For this review, take the finished solid that the model builds, in its own axes (mm). A direction names the side the tool comes from. Give positions to 0.01 mm unless a question says otherwise; leave off trailing zeros.
Q1. Machinability: for faces 4 (the cylindrical face through (0.54, 7.56, 1.68)), 5 (the flat face through (-8, 12.845, 6)), 6 (the flat face through (2.655, 2, 6)), which of the approach directions +Z, -Z, +X, -X, +Y, -Y give a long, thin tool a straight path to every point of the face, cutting with its end or side? Answer none if there is none.
Q2. Mouldability with a two-part tool opening along Y and no side actions: class faces 1 (the flat face through (4.13, 14.03, 5.88)), 2 (the flat face through (-2.845, 2, 6)), 3 (the flat face through (4, 0, 3)) as released by +Y, released by -Y, zero draft, split by the parting line, or undercut.
Q3. Insertion check: P1, Ø4, axis at x = 50, y = 9.5, coming from the +Z side; P2, Ø3.5, axis at y = 3, z = 6, coming from the -X side; P3, Ø3, axis at x = 76, z = 2.5, coming from the -Y side; P4, Ø4, axis at x = 60, z = 4, coming from the +Y side. Each pin has a flat end and moves straight along its axis. Give the tip position at first contact, or say it passes through.
Q4. We need section A-A (z = 5.5). Give the number of separate pieces and of enclosed holes in the cut face, then the cut area to 3 significant figures.
Q5. For line 1 (Y direction, x = 0, z = 1.45); line 2 (Y direction, x = 0, z = 3.65); line 3 (Z direction, x = 0, y = 3.5), list the stretches that pass through material, from the lowest coordinate up.
```python
from build123d import *

# Parameters (mm, degrees)
BOSS_EXTRU_1_DEPTH       = 8
ESQUISSE13_R             = 4
ENL_V_MAT_EXTRU_9_DEPTH  = 4.3
ENL_V_MAT_EXTRU_10_DEPTH = 4.3
ESQUISSE15_R             = 2.5
ENL_V_MAT_EXTRU_11_DEPTH = 3.4
ENL_V_MAT_EXTRU_12_REACH = 113.898
ESQUISSE16_R             = 1.25
ESQUISSE17_OUTSIDE_W     = 146.384
ESQUISSE17_OUTSIDE_H     = 46.384
ENL_V_MAT_EXTRU_13_DEPTH = 10
ENL_V_MAT_EXTRU_14_DEPTH = 10


with BuildPart() as part:
    # Esquisse1 → Boss.-Extru.1 (new body)
    with BuildSketch(Plane.XY):
        with BuildLine():
            Line((0, 0), (100, 0))
            ThreePointArc((100, 0), (110, 10), (100, 20))
            Line((100, 20), (0, 20))
            ThreePointArc((0, 20), (-10, 10), (0, 0))
        make_face()
    extrude(amount=BOSS_EXTRU_1_DEPTH)

    # Esquisse13 → Enlèv. mat.-Extru.9 (cut)
    with BuildSketch(Plane.XY.offset(8)):
        with Locations((0, 10)):
            Circle(ESQUISSE13_R)
    extrude(amount=-ENL_V_MAT_EXTRU_9_DEPTH, mode=Mode.SUBTRACT)

    # Esquisse14 → Enlèv. mat.-Extru.10 (cut)
    with BuildSketch(Plane.XY.offset(8)):
        Polygon((2.655377087, 4.544050257), (2.655377087, -2.008601379), (-2.844622913, -1.912365766), (-2.844622913, 4.640285869), (-5.455949743, 7.344622913), (-12.008601379, 7.344622913), (-11.912365766, 12.844622913), (-5.359714131, 12.844622913), (-2.655377087, 15.455949743), (-2.655377087, 22.008601379), (2.844622913, 21.912365766), (2.844622913, 15.359714131), (5.455949743, 12.655377087), (12.008601379, 12.655377087), (17.818097103, 12.655377087), (17.818097103, 7.155377087), (11.912365766, 7.155377087), (5.359714131, 7.155377087), align=None)
    extrude(amount=-ENL_V_MAT_EXTRU_10_DEPTH, mode=Mode.SUBTRACT)

    # Esquisse15 → Enlèv. mat.-Extru.11 (cut)
    with BuildSketch(Plane(origin=(0, 0, 0), x_dir=(-1, 0, 0), z_dir=(0, 0, -1))):
        with Locations((0, 10)):
            Circle(ESQUISSE15_R)
    extrude(amount=-ENL_V_MAT_EXTRU_11_DEPTH, mode=Mode.SUBTRACT)

    # Esquisse16 → Enlèv. mat.-Extru.12 (cut, up to next)
    with BuildSketch(Plane(origin=(0, 0, 3.4), x_dir=(-1, 0, 0), z_dir=(0, 0, -1)), mode=Mode.PRIVATE) as enl_v_mat_extru_12_sk1:
        with Locations((0, 10)):
            Circle(ESQUISSE16_R)
    enl_v_mat_extru_12_tool1 = extrude(enl_v_mat_extru_12_sk1.sketch, amount=-ENL_V_MAT_EXTRU_12_REACH, mode=Mode.PRIVATE) & part.part
    add(enl_v_mat_extru_12_tool1.solids().sort_by_distance((0, 10, 3.4))[0], mode=Mode.SUBTRACT)

    # Esquisse17 outside → Enlèv. mat.-Extru.13 (cut)
    with BuildSketch(Plane.XY.offset(8)):
        with Locations((50, 10)):
            Rectangle(ESQUISSE17_OUTSIDE_W, ESQUISSE17_OUTSIDE_H)
        with BuildLine():
            add(Edge.make_bspline(
                [(6.078713642, 20), (24.915023514, 16.081550404), (43.772946516, 24.459557565), (129.172588167, 9.95529611), (44.539574838, -4.288408378), (17.569235721, 5.732265476), (-18.329346207, -7.417520102), (-23.15173951, 28.634629281), (-5.183949024, 22.342931088), (6.078713642, 20)],
                knots=[0, 0, 0, 0, 0.182524448, 0.382167519, 0.581810591, 0.764335038, 0.867297941, 0.890864437, 1, 1, 1, 1], degree=3))
        make_face(mode=Mode.SUBTRACT)
    extrude(amount=-ENL_V_MAT_EXTRU_13_DEPTH, mode=Mode.SUBTRACT)

    # Esquisse18 → Enlèv. mat.-Extru.14 (cut)
    with BuildSketch(Plane.XY.offset(8)):
        Polygon((13.616328718, 4.640285869), (13.71095163, 15.455949743), (90.655144278, 10.048117806), align=None)
    extrude(amount=-ENL_V_MAT_EXTRU_14_DEPTH, mode=Mode.SUBTRACT)


solid = part.part
```
Computed:
1. face 4: -Z
1. face 5: +Z, -X
1. face 6: +Z, +Y, -Y
2. face 1: undercut
2. face 2: zero draft
2. face 3: released by -Y
3. P1: passes through
3. P2: stops at x = -8.51
3. P3: stops at y = 1.81
3. P4: stops at y = 19.8
4. separate pieces: 3
4. enclosed holes: 0
4. area: 1,180 mm2
5. line 1: y = 0 to 7.5, 12.5 to 20
5. line 2: y = 0 to 8.75, 11.25 to 20
5. line 3: z = 0 to 3.7
